Autodesk Inventor part; units mm, degrees
ref_plane "РабПлоскость1" through (0, -23.25, 0) normal (0, -1, 0) x (1, 0, 0)
ref_plane "РабПлоскость2" through (1, 3, -27.6612) normal (0, 1, 0) x (1, 0, 0)
ref_plane "YZ Plane" through (0, 0, 0) normal (1, 0, 0) x (0, 1, 0)
sketch "Эскиз1" plane through (0, 0, 0) normal (0, 1, 0) x (-1, 0, 0)
  point P0 (0, 0)
sketch "Эскиз2" plane through (0, 0, 0) normal (0, 1, 0) x (-1, 0, 0)
  line L0 (0, 0) -> (0, -68)
  line L1 (0, -68) -> (-10, -68)
  line L2 (-10, -68) -> (-10, -48)
  line L3 (-10, -48) -> (-40, -48)
  line L4 (0, 0) -> (-10, 0)
  line L5 (-10, 0) -> (-10, -5)
  line L6 (-40, -48) -> (-40, -34)
  line L7 (-40, -34) -> (-10, -5)
  dimension "d0" = 68
  dimension "d1" = 10
  dimension "d2" = 20
  dimension "d3" = 30
  dimension "d4" = 5
  dimension "d5" = 14
extrude "Выдавливание1" add sketch "Эскиз2" along normal blind 28
sketch "Эскиз3" plane through (0, 0, -68) normal (-1, 0, 0) x (0, 0, 1)
  line L0 (68, 0) -> (68, 28)
  line L1 (68, 14) -> (33, 14)
  arc A0 (40, 0) -> (40, 28) centre (50.5, 14) ccw
  line L2 (0, 0) -> (68, 0)
  line L3 (40, 0) -> (0, 0)
  line L4 (20, 28) -> (0, 28)
  line L5 (0, 0) -> (0, 28)
  line L6 (0, 28) -> (40, 28)
  line L7 (0, 28) -> (68, 28)
  dimension "d8" = 35
extrude "Выдавливание2" add sketch "Эскиз3" against normal blind 40 contours A0 L2 L5 L4 L6 L7 | A0 L2 | L7 A0
ref_plane "РабПлоскость1" through (0, -23.25, 0) normal (0, -1, 0) x (1, 0, 0)
sketch "Эскиз4" plane through (0, -23.25, 0) normal (0, -1, 0) x (1, 0, 0)
  line L0 (0, -68) -> (40, -68)
  line L1 (0, -68) -> (10, -68)
  line L2 (10, -68) -> (10, -48)
  line L3 (10, -48) -> (40, -48)
  line L4 (40, -48) -> (40, -34)
  line L5 (10, 0) -> (10, -5)
  line L6 (40, -34) -> (10, -5)
  line L7 (0, 0) -> (10, 0)
  line L8 (10, -5) -> (10, 0)
  line L9 (10, 0) -> (0, 0)
  line L10 (0, 0) -> (0, -68)
  dimension "d12" = 10
  dimension "d13" = 20
  dimension "d14" = 30
  dimension "d15" = 14
extrude "Выдавливание3" cut sketch "Эскиз4" against normal blind 139 keep common part
sketch "Эскиз5" plane through (0, 0, 0) normal (-1, 0, 0) x (0, 0, 1)
  arc A0 (-28, 0) -> (-7, 0) centre (-17.5, 14) ccw
  circle A1 centre (-17.5, 14) radius 17.5
  line L0 (-68, 0) -> (-68, 28)
  line L1 (-28, 0) -> (-68, 0)
  line L2 (-68, 0) -> (-68, 28)
  arc A2 (-7, 28) -> (-28, 28) centre (-17.5, 14) ccw
  line L3 (-68, 28) -> (-28, 28)
  point P0 (0, 0)
extrude "Выдавливание4" cut sketch "Эскиз5" against normal blind 43.75 keep common part
sketch "Эскиз6" plane through (40, 0, -34) normal (1, 0, 0) x (0, 0, -1)
  arc A0 (-29, 1.7526) -> (-6, 0) centre (-16.5, 14) ccw
  circle A1 centre (-16.5, 14) radius 16.5
  line L0 (0, 0) -> (0, 28)
  line L1 (0, 14) -> (34.1975, 14)
  line L2 (34, 28) -> (-6, 28)
  line L3 (34, 0) -> (-6, 0)
  line L4 (34, 28) -> (34, 0)
  line L5 (34, 0) -> (34, 28)
  line L6 (34, 28) -> (34, 27)
  line L7 (34, 27) -> (-6.3388, 27)
  line L8 (34, 0) -> (34, 1)
  line L9 (34, 1) -> (-6.3388, 1)
  line L10 (34, 27) -> (-6.3388, 27)
  line L11 (34, 27) -> (34, 1)
  point P0 (-34, 0)
  point P1 (0, 27)
  dimension "d20" = 33
  dimension "d21" = 1
  dimension "d22" = 1
extrude "Выдавливание5" cut sketch "Эскиз6" against normal blind 39 contours A1 | L0 L9 A1 | L1 L4 L9 L0 | A1 L7 L0 | L0 L7 L4 L1
fillet "Сопряжение1" radius 8 2 edges at (40, 0.5, -48) (40, 27.5, -48)
fillet "Сопряжение2" radius 8 2 edges at (40, 0.5, -34) (40, 27.5, -34)
fillet "Сопряжение3" radius 8 2 edges at (10, 0.5, -68) (10, 27.5, -68)
sketch "Эскиз7" plane through (0, 28, 0) normal (0, 1, 0) x (1, 0, 0)
  arc A0 (40, 40) -> (32, 48) centre (32, 40) ccw
  circle A1 centre (32, 40) radius 3
  point P0 (0, 0)
  dimension "d28" = 6
extrude "Выдавливание6" add sketch "Эскиз7" along normal blind 4 and the other way blind 32
sketch "Эскиз8" plane through (1, 0, -34) normal (1, 0, 0) x (0, 0, -1)
  arc A0 (-6.3388, 27) -> (-29, 24.7703) centre (-16.5, 14) ccw
  circle A1 centre (-16.5, 14) radius 5
  point P0 (-34, 0)
  dimension "d31" = 10
extrude "Выдавливание7" cut sketch "Эскиз8" against normal blind 31
ref_plane "РабПлоскость2" through (1, 3, -27.6612) normal (0, 1, 0) x (1, 0, 0)
sketch "Эскиз9" plane through (1, 3, -27.6612) normal (0, 1, 0) x (1, 0, 0)
  circle A0 centre (31, 12.3388) radius 3
  circle A1 centre (31, 12.3388) radius 25
  point P0 (-1, -27.6612)
  dimension "d35" = 50
extrude "Выдавливание8" add sketch "Эскиз9" along normal blind 22
fillet "Сопряжение4" radius 8 2 edges at (7, 3, -40) (7, 25, -40)
chamfer "Фаска1" distance 1 angle 45 2 edges at (29, -4, -40) (29, 32, -40)
properties part number "Колесо"
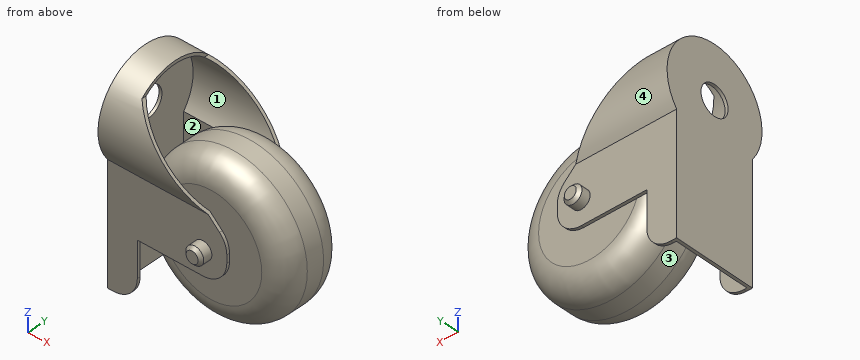
Here's how the part is built. I have some questions about the finished solid (model axes, mm). Face numbers are marked on the shaded views. A direction names the side the tool comes from. Round coordinates to 2 decimals unless told otherwise and drop trailing zeros. Write each loop counter-clockwise with the first axis right and the second up, starting at its lowest first coordinate (ties: lowest second). Pieces come first, ordered by that corner, then holes.
Q1. Please list where these lines run through material, in increasing order: probe 1 along Y at (x, z) = (8.5, -17.5); probe 2 along Y at (x, z) = (0.45, -17.5); probe 3 along Y at (x, z) = (34.5, -29).
Q2. Which directions (+Z, -Z, +X, -X, +Y, -Y) give clear straight access to the entire face, cutting with the end or side of a thin tool? Please do the marked faces 3 and 4.
Q3. If we section it at A-A on y = 14: Write out the boundary of the cut face in (x, z), plus the area to 3 significant figures.
Q4. If we section it at B-B on y = 5.5: Write out the boundary of the cut face in (x, z), plus the area to 3 significant figures.
Q5. Will these pins go through, and if not, where does the flat tip stop? P1, Ø12, axis at x = 28.5, z = -54.5, coming from the -Y side; P2, Ø2, axis at x = 51, z = -32, coming from the +Y side; P3, Ø1.1, axis at y = 27.5, z = -55.5, coming from the +X side; P4, Ø3, axis at y = 21, z = -31.5, coming from the -X side.
Q6. If we mould it in two halves opening along Z, with no side actions, what happens to the marked faces 1 and 2? For each: +Z half, -Z half, draft (parallel to the pull), parting line (faces both ways), or undercut.
Q7. If we section it at C-C on z = -11.5: Write out the boundary of the cut face in (x, y).
Answer below:
1. probe 1: y = -3.5 to -2.5, 30.5 to 31.5
1. probe 2: y = -3.5 to 9, 19 to 31.5
1. probe 3: y = 0 to 1, 3 to 25, 27 to 28
2. face 3: none
2. face 4: +X, -X
3. outline: (0, -68) - (1, -68) - (1, -22.5) - (0, -22.5) - close; (0, -12.5) - (1, -12.5) - (1, -1) - (10, -1) - (10, 0) - (0, 0) - close; circle Ø50 at (32, -40)
3. area: 2,030 mm2
4. outline: (0, -68) - (1, -68) - (1, -3.36) - (10, -3.36) - (10, -2.2) - (0, -2.2) - close; circle Ø45.62 at (32, -40)
4. area: 1,710 mm2
5. P1: stops at y = 3
5. P2: stops at y = 24.56
5. P3: stops at x = 10
5. P4: stops at x = 0
6. face 1: undercut
6. face 2: draft
7. outline: (0, -2.44) - (16.72, -2.44) - (16.72, -1.37) - (1, -1.37) - (1, 29.37) - (16.72, 29.37) - (16.72, 30.44) - (0, 30.44) - close
